Design review of the part built by this model. Coordinates are the model's own, in mm. A direction names the side the tool comes from. Give positions to 0.01 mm unless a question says otherwise; leave off trailing zeros. Loops run counter-clockwise (first coordinate to the right, second up) from the corner with the lowest first, then second, coordinate; pieces in that order, holes last. Notation, with made-up numbers: (84, 55.25) -> (131, 55.25) arc R24 cw to (131, 90.25) -> close; hole circle Ø4 at (23.5, 34.5). An arc over 180 degrees is marked (long way). Use CSV: the item, a comma, the result in double quotes. Start each with the question number.
Item 1: We need section B-B (x = 37.5). State the section outline as (y, z) points, plus the area to 3 significant figures.
Item 2: For faces 5 (the face through (15.26, -2.788, 5.517)), 6 (the face through (25, -37, 7)), 7 (the face through (17.5, -7, 8)), 8 (the face through (70, -28, 7)), list the 3-axis set-ups (+Z, -Z, +X, -X, +Y, -Y) from which the entire face can be reached by the end or side of a thin tool; tool diameter is ignored.
Item 3: Clearance check with flat-ended pins moving along their axes: pin 1 (4.5 mm diameter, centred on y = -27, z = 8, fed in from -X); pin 2 (3.5 mm diameter, centred on x = 15, z = 7.5, fed in from +Y); pin 3 (1.8 mm diameter, centred on x = 60, y = -37, fed in from -Z); pin 4 (2 mm diameter, centred on y = -6.5, z = 7, fed in from +X). State where each tip first meets the part, or that it passes through.
Item 4: We need section C-C (z = 3.5). State the section outline as (x, y) points.
Item 5: Wall thickness on line 1 along Y through (x, z) = (26, 12.5); line 2 along X through (y, z) = (-34.5, 11.25); line 3 along X through (y, z) = (-3.9, 7.5): over which ranges is each line inside the solid? List them lowest first. Write a range as from..to.
Item 6: We need section A-A (z = 7.5). State the section outline as (x, y) points.
Item 7: We need section D-D (y = -22). State the section outline as (x, z) points, plus the area to 3 significant figures.
Item 8: The part is to be moulded in two halves that separate along X. For faces 1 (the face through (16.233, -6.768, 9.675)), 2 (the face through (0, -5, 7)), 3 (the face through (63.986, -5.703, 7.395)), 4 (the face through (51, -23, 15)), say which applies: +X half, -X half, draft (parallel to the pull), parting line (faces both ways), or undercut.
from build123d import *

# Parameters (mm, degrees)
ESQUISSE1_R             = 1.5
BOSS_EXTRU_1_DEPTH      = 15
ESQUISSE3_R             = 5
ENL_V_MAT_EXTRU_1_DEPTH = 2
ESQUISSE4_R             = 2
ENL_V_MAT_EXTRU_2_DEPTH = 9
ENL_V_MAT_EXTRU_3_DEPTH = 2.5


with BuildPart() as part:
    # Esquisse1 → Boss.-Extru.1 (new body)
    with BuildSketch(Plane.XY):
        with BuildLine():
            Line((0, 0), (50, 0))
            ThreePointArc((50, 0), (64.142135624, -5.857864376), (70, -20))
            Line((70, -20), (70, -37))
            ThreePointArc((70, -37), (67.071067812, -44.071067812), (60, -47))
            Line((60, -47), (0, -47))
            Line((0, -47), (0, -37))
            Line((0, -37), (50, -37))
            Line((50, -37), (50, -10))
            Line((50, -10), (0, -10))
            Line((0, -10), (0, 0))
        make_face()
        with Locations((60, -37)):
            Circle(ESQUISSE1_R, mode=Mode.SUBTRACT)
    extrude(amount=BOSS_EXTRU_1_DEPTH)

    # Esquisse3 → Enlèv. mat.-Extru.1 (cut)
    with BuildSketch(Plane.XZ.offset(10)):
        with Locations((15, 7.5)):
            Circle(ESQUISSE3_R)
    extrude(amount=-ENL_V_MAT_EXTRU_1_DEPTH, mode=Mode.SUBTRACT)

    # Esquisse4 → Enlèv. mat.-Extru.2 (cut, through all)
    with BuildSketch(Plane(origin=(0, -8, 0), x_dir=(-1, 0, 0), z_dir=(0, -1, 0))):
        with Locations((-15, -7.5)):
            Circle(ESQUISSE4_R)
    extrude(amount=-ENL_V_MAT_EXTRU_2_DEPTH, mode=Mode.SUBTRACT)

    # Esquisse5 → Enlèv. mat.-Extru.3 (cut)
    with BuildSketch(Plane.XZ.offset(8)):
        Polygon((12.5, 6.056624327), (12.5, 8.943375673), (15, 10.386751346), (17.5, 8.943375673), (17.5, 6.056624327), (15, 4.613248654), align=None)
    extrude(amount=-ENL_V_MAT_EXTRU_3_DEPTH, mode=Mode.SUBTRACT)


solid = part.part
Results found:
1,outline,"(-47, 0) -> (-37, 0) -> (-37, 15) -> (-47, 15) -> close; (-10, 0) -> (0, 0) -> (0, 15) -> (-10, 15) -> close"
1,area,"300 mm²"
2,face 5,"+Y"
2,face 6,"+Z, -Z, -X"
2,face 7,"none"
2,face 8,"+Z, -Z, +X, +Y, -Y"
3,pin 1,"x = 50"
3,pin 2,"y = -37"
3,pin 3,"through"
3,pin 4,"x = 65.61"
4,outline,"(0, -47) -> (60, -47) arc R10 ccw to (70, -37) -> (70, -20) arc R20 ccw to (50, 0) -> (0, 0) -> (0, -10) -> (12, -10) -> (12, -8) -> (18, -8) -> (18, -10) -> (50, -10) -> (50, -37) -> (0, -37) -> close; hole circle Ø3 at (60, -37)"
5,line 1,"-47..-37, -10..0"
5,line 2,"50..70"
5,line 3,"0..13, 17..61.87"
6,outline,"(0, -47) -> (60, -47) arc R10 ccw to (70, -37) -> (70, -20) arc R20 ccw to (50, 0) -> (17, 0) -> (17, -5.5) -> (17.5, -5.5) -> (17.5, -8) -> (20, -8) -> (20, -10) -> (50, -10) -> (50, -37) -> (0, -37) -> close; (0, -10) -> (10, -10) -> (10, -8) -> (12.5, -8) -> (12.5, -5.5) -> (13, -5.5) -> (13, 0) -> (0, 0) -> close; hole circle Ø3 at (60, -37)"
7,outline,"(50, 0) -> (70, 0) -> (70, 15) -> (50, 15) -> close"
7,area,"300 mm²"
8,face 1,"undercut"
8,face 2,"-X half"
8,face 3,"+X half"
8,face 4,"draft"
